from build123d import *

# Parameters (mm, degrees)
SKETCH_1_W                  = 12.8
SKETCH_1_H                  = 22.2
EXTRUDE_1_DEPTH             = 10
SKETCH_3_W                  = 4
SKETCH_3_H                  = 4
CUT_EXTRUDE_1_DEPTH         = 6.4
PATTERN_LINEAR_1_COUNT      = 5
PATTERN_LINEAR_1_PITCH      = 4.2
PATTERN_LINEAR_1_COUNT_DIR2 = 2
PATTERN_LINEAR_1_PITCH_DIR2 = 4.2
SKETCH_12_W                 = 1
SKETCH_12_H                 = 1
CUT_EXTRUDE_2_DEPTH         = 6.4
PATTERN_LINEAR_2_COUNT      = 5
PATTERN_LINEAR_2_PITCH      = 4.2
PATTERN_LINEAR_2_COUNT_DIR2 = 2
PATTERN_LINEAR_2_PITCH_DIR2 = 4.2
SKETCH_14_W                 = 1
SKETCH_14_H                 = 1
SKETCH_16_W                 = 1
SKETCH_16_H                 = 1
PATTERN_LINEAR_3_COUNT      = 5
PATTERN_LINEAR_3_PITCH      = 4.2
SKETCH_18_W                 = 3
SKETCH_18_H                 = 3.2
EXTRUDE_2_DEPTH             = 1.5
CUT_EXTRUDE_3_DEPTH         = 3.2


with BuildPart() as part:
    # Эскиз1 → Бобышка-Вытянуть1 (new body)
    with BuildSketch(Plane(origin=(0, 0, 0), x_dir=(1, 0, 0), z_dir=(0, 1, 0))):
        Rectangle(SKETCH_1_W, SKETCH_1_H)
    extrude(amount=EXTRUDE_1_DEPTH)

    # Эскиз3 → Вырез-Вытянуть1 (cut)
    with BuildSketch(Plane.ZY.offset(6.4)):
        with Locations((-8.4, 7.1)):
            Rectangle(SKETCH_3_W, SKETCH_3_H)
    cut_extrude_1 = extrude(amount=-CUT_EXTRUDE_1_DEPTH, mode=Mode.SUBTRACT)

    # Линейный массив1: Cut-Extrude 1 5 × 2
    with Locations(*[(0, -j * PATTERN_LINEAR_1_PITCH_DIR2, i * PATTERN_LINEAR_1_PITCH) for i in range(PATTERN_LINEAR_1_COUNT) for j in range(PATTERN_LINEAR_1_COUNT_DIR2) if (i, j) != (0, 0)]):
        add(cut_extrude_1, mode=Mode.SUBTRACT)

    # Эскиз12 → Вырез-Вытянуть2 (cut)
    with BuildSketch(Plane(origin=(6.4, 0, 0), x_dir=(0, 0, -1), z_dir=(1, 0, 0))):
        with Locations((-8.4, 7.1)):
            Rectangle(SKETCH_12_W, SKETCH_12_H)
    cut_extrude_2 = extrude(amount=-CUT_EXTRUDE_2_DEPTH, mode=Mode.SUBTRACT)

    # Линейный массив2: Cut-Extrude 2 5 × 2
    with Locations(*[(0, -j * PATTERN_LINEAR_2_PITCH_DIR2, -i * PATTERN_LINEAR_2_PITCH) for i in range(PATTERN_LINEAR_2_COUNT) for j in range(PATTERN_LINEAR_2_COUNT_DIR2) if (i, j) != (0, 0)]):
        add(cut_extrude_2, mode=Mode.SUBTRACT)

    # По траектории6: sweep along a path in Эскиз15
    with BuildLine(Plane.XY.offset(11.1)) as sweep_6_path:
        Line((-3, 7.1), (12.1, 7.1))
        ThreePointArc((12.1, 7.1), (12.807106781, 6.807106781), (13.1, 6.1))
        Line((13.1, 6.1), (13.1, -3.5))
    # Эскиз14 → По траектории6 (sweep)
    with BuildSketch(Plane(origin=(0, -3.5, 0), x_dir=(1, 0, 0), z_dir=(0, 1, 0))):
        with Locations((13.1, -8.4)):
            Rectangle(SKETCH_14_W, SKETCH_14_H)
    sweep_6 = sweep(path=sweep_6_path.line)

    # По траектории7: sweep along a path in Эскиз17
    with BuildLine(Plane.XY.offset(11.1)) as sweep_7_path:
        Line((7.6, -3.5), (7.6, 1.9))
        ThreePointArc((7.6, 1.9), (7.307106781, 2.607106781), (6.6, 2.9))
        Line((6.6, 2.9), (-3, 2.9))
    # Эскиз16 → По траектории7 (sweep)
    with BuildSketch(Plane(origin=(0, -3.5, 0), x_dir=(1, 0, 0), z_dir=(0, 1, 0))):
        with Locations((7.6, -8.4)):
            Rectangle(SKETCH_16_W, SKETCH_16_H)
    sweep_7 = sweep(path=sweep_7_path.line)

    # Линейный массив3: По траектории6, По траектории7 ×5
    with Locations(*[(0, 0, -i * PATTERN_LINEAR_3_PITCH) for i in range(1, PATTERN_LINEAR_3_COUNT)]):
        add(sweep_6)
        add(sweep_7)

    # Эскиз18 → Бобышка-Вытянуть2 (add)
    with BuildSketch(Plane(origin=(0, 10, 0), x_dir=(1, 0, 0), z_dir=(0, 1, 0))):
        with Locations((-4.9, 0)):
            Rectangle(SKETCH_18_W, SKETCH_18_H)
    extrude(amount=EXTRUDE_2_DEPTH)

    # Эскиз19 → Вырез-Вытянуть3 (cut)
    with BuildSketch(Plane.XY.offset(1.6)):
        Polygon((-3.4, 11.5), (-6.4, 10), (-6.4, 11.5), align=None)
    extrude(amount=-CUT_EXTRUDE_3_DEPTH, mode=Mode.SUBTRACT)


solid = part.part
Read the model definition and answer for the solid it produces. Units are mm, in the model's axes. A direction names the side the tool comes from. Give positions to 0.01 mm unless a question says otherwise; leave off trailing zeros. Write each loop counter-clockwise with the first axis right and the second up, starting at its lowest first coordinate (ties: lowest second). Pieces come first, ordered by that corner, then holes. Notation, with made-up numbers: (51, 87.25) - (62, 87.25) arc R8 ccw to (62, 92.25) - close; hole circle Ø1 at (76, -3.75). An arc over 180 degrees is marked (long way). Use CSV: the item, a comma, the result in double quotes. Start each with the question number.
Item 1: For faces 1 (the flat face through (9, 6.6, 4)), 2 (the flat face through (-3, 3, -2)), 3 (the flat face through (7.5, 0, 3.7)), determine the directions among +Z, -Z, +X, -X, +Y, -Y from which every point of the face is accessible in a straight line to the end or side of a thin tool.
Item 2: The part is cut by section B-B, the plane y = 8. Give the vertices of the cut face in (x, z).
Item 3: Flat-ended cylindrical pins translate along their axes: P1, Ø1.2, axis at x = -3.5, z = 0.5, coming from the -Y side; P2, Ø4, axis at x = -4, z = -6, coming from the +Y side; P3, Ø1.1, axis at y = -1, z = -8.5, coming from the -X side. Find the tip coordinate at first contact, or state that the pin passes through.
Item 4: Consider line 1 (Y direction, x = -0.25, z = -8.5); line 2 (Y direction, x = -1.75, z = 3); line 3 (Z direction, x = -5.5, y = 4.5). Determine where each line is inside the solid, lowest interval first.
Item 5: The mould has two halves that part along Z. Classify faces 4 (the flat face through (-1.5, 2.4, -8.4)), 5 (the flat face through (13, 3, 8.9)), 6 (the flat face through (9, 7.6, 0)): pulls with the +Z half, pulls with the -Z half, needs draft (parallel to the pull), parting line crosses it, or undercut.
Item 6: The part is cut by section D-D, the plane x = -5. Count the separate pieces of the cut face and the enclosed holes in it, and give its area (3 significant figures).
Item 7: The part is cut by section C-C, the plane z = 7. Give the vertices of the cut face in (x, y), and give its area (3 significant figures).
Item 8: The part is cut by section A-A, the plane x = 8.75. Give the vertices of the cut face in (y, z).
Taken from the geometry:
1,face 1,"+Z, -Z"
1,face 2,"-X"
1,face 3,"+X, +Y, -Y"
2,outline,"(-6.4, -11.1) - (6.4, -11.1) - (6.4, 11.1) - (-6.4, 11.1) - (-6.4, 10.4) - (0, 10.4) - (0, 6.4) - (-6.4, 6.4) - (-6.4, 6.2) - (0, 6.2) - (0, 2.2) - (-6.4, 2.2) - (-6.4, 2) - (0, 2) - (0, -2) - (-6.4, -2) - (-6.4, -2.2) - (0, -2.2) - (0, -6.2) - (-6.4, -6.2) - (-6.4, -6.4) - (0, -6.4) - (0, -10.4) - (-6.4, -10.4) - close"
3,P1,"y = 0"
3,P2,"y = 10"
3,P3,"x = 7.1"
4,line 1,"0 to 0.9, 2.4 to 3.4, 4.9 to 5.1, 6.6 to 7.6, 9.1 to 10"
4,line 2,"0 to 0.9, 4.9 to 5.1, 9.1 to 10"
4,line 3,"-11.1 to -10.4, -6.4 to -6.2, -2.2 to -2, 2 to 2.2, 6.2 to 6.4, 10.4 to 11.1"
5,face 4,"undercut"
5,face 5,"pulls with the +Z half"
5,face 6,"needs draft"
6,separate pieces,"1"
6,enclosed holes,"10"
6,area,"64.2 mm2"
7,outline,"(-6.4, 0) - (6.4, 0) - (6.4, 10) - (-6.4, 10) - (-6.4, 9.1) - (0, 9.1) - (0, 5.1) - (-6.4, 5.1) - (-6.4, 4.9) - (0, 4.9) - (0, 0.9) - (-6.4, 0.9) - close"
7,area,"76.8 mm2"
8,outline,"(6.6, -8.9) - (7.6, -8.9) - (7.6, -7.9) - (6.6, -7.9) - close; (6.6, -4.7) - (7.6, -4.7) - (7.6, -3.7) - (6.6, -3.7) - close; (6.6, -0.5) - (7.6, -0.5) - (7.6, 0.5) - (6.6, 0.5) - close; (6.6, 3.7) - (7.6, 3.7) - (7.6, 4.7) - (6.6, 4.7) - close; (6.6, 7.9) - (7.6, 7.9) - (7.6, 8.9) - (6.6, 8.9) - close"
